Source: CAD feature listing. Evaluate the final solid. Frame: model axes, mm. A direction names the side the tool comes from. Coordinates: 2 decimals unless noted, no trailing zeros. Write each loop counter-clockwise with the first axis right and the second up, starting at its lowest first coordinate (ties: lowest second). Pieces come first, ordered by that corner, then holes. Notation, with made-up numbers: (43, 61) - (52, 61) arc R28 cw to (52, 89) - close; hole circle Ø1 at (24, 78.25). An arc over 180 degrees is marked (long way). One line per item, written item: value.
Autodesk Inventor part; units mm, degrees
ref_plane "Work Plane6" through (4.5, 0, 0) normal (1, 0, 0) x (0, 1, 0)
ref_plane "Work Plane7" through (0, -17.5, 0) normal (0, 1, 0) x (-1, 0, 0)
ref_plane "Work Plane8" through (0, 0, 15.25) normal (0, 0, 1) x (1, 0, 0)
sketch "Sketch1" plane through (0, 0, 0) normal (0, 0, 1) x (1, 0, 0)
  line L0 (-41.267, 50.1755) -> (50.733, 50.1755)
  line L1 (50.733, 50.1755) -> (50.733, -91.8245)
  line L2 (50.733, -91.8245) -> (-41.267, -91.8245)
  line L3 (-41.267, -91.8245) -> (-41.267, 50.1755)
  point P0 (0, 0)
  dimension "d0" = 142
  dimension "d1" = 92
extrude "Extrusion1" add sketch "Sketch1" along normal blind 14
sketch "Sketch2" plane through (0, 0, 14) normal (0, 0, 1) x (1, 0, 0)
  line L0 (50.733, 50.1755) -> (-41.267, 50.1755)
  line L1 (-41.267, -91.8245) -> (50.733, -91.8245)
  line L2 (50.733, -91.8245) -> (50.733, 50.1755)
  line L3 (50.733, 50.1755) -> (-41.267, 50.1755)
  line L4 (-41.267, 50.1755) -> (-41.267, -91.8245)
  circle A0 centre (29.733, 34.3976) radius 9
  circle A1 centre (-20.267, 34.3976) radius 9
  circle A2 centre (-20.267, -65.6024) radius 9
  circle A3 centre (29.733, -65.6024) radius 9
  point P0 (0, 0)
  point P1 (-20.267, 50.1755)
  point P2 (29.733, 50.1755)
  point P3 (50.733, 29.1755)
  point P4 (-41.267, 29.1755)
  point P5 (-41.267, 29.1755)
  point P6 (-20.267, 50.1755)
  point P7 (50.733, 29.1755)
  dimension "d5" = 21
  dimension "d6" = 21
  dimension "d7" = 50
  dimension "d8" = 21
  dimension "d9" = 21
  dimension "d13" = 18
  dimension "d14" = 18
  dimension "d15" = 100
  dimension "d16" = 100
  dimension "d17" = 18
  dimension "d18" = 18
extrude "Extrusion2" cut sketch "Sketch2" against normal through all contours A0 | A1 | A2 | A3
sketch "Sketch3" plane through (0, 0, 14) normal (0, 0, 1) x (1, 0, 0)
  circle A0 centre (-20.267, 34.3976) radius 9
  circle A1 centre (29.733, 34.3976) radius 9
  line L0 (50.733, -91.8245) -> (50.733, 50.1755)
  line L1 (-41.267, 50.1755) -> (-41.267, -91.8245)
  line L2 (50.733, -8.1024) -> (-41.267, -8.1024)
  line L3 (-41.267, -8.1024) -> (-41.267, -26.6259)
  line L4 (-41.267, -26.6259) -> (50.733, -26.6259)
  line L5 (50.733, -26.6259) -> (50.733, -8.1024)
  point P0 (0, 0)
  point P1 (-20.267, -8.1024)
  point P2 (31.8821, -8.1024)
  point P3 (50.733, -81.8245)
  point P4 (50.733, 40.1755)
  point P5 (-41.267, 40.1755)
  point P6 (-41.267, -81.8245)
  dimension "d22" = 42.5
  dimension "d23" = 42.5
  dimension "d54" = 92
  dimension "d55" = 92
extrude "Extrusion5" add sketch "Sketch3" along normal blind 58 contours L4 L1 L2 L0
chamfer "Chamfer1" distance 36 angle 45 2 edges at (50.733, -17.3641, 72) (-41.267, -17.3641, 72)
sketch "Sketch10" plane through (-41.267, -8.1024, 14) normal (0, 1, 0) x (1, 0, 0)
  line L0 (92, 0) -> (92, -22)
  line L1 (0, 0) -> (92, 0)
  point P0 (41.267, 14)
sketch "Sketch11" plane through (-41.267, -26.6259, 14) normal (0, -1, 0) x (1, 0, 0)
  line L0 (92, 0) -> (0, 0)
  line L1 (36, 58) -> (56, 58)
  point P0 (41.267, -14)
  point P1 (46, 58)
  point P2 (46, 0)
  dimension "d64" = 46
  dimension "d65" = 46
ref_plane "Work Plane6" through (4.5, 0, 0) normal (1, 0, 0) x (0, 1, 0)
sketch "Sketch12" plane through (4.5, 0, 0) normal (1, 0, 0) x (0, 1, 0)
  line L0 (-8.1024, 14) -> (32.8976, 14)
  line L1 (-8.1024, 14) -> (-8.1024, 72)
  line L2 (-8.1024, 72) -> (32.8976, 14)
  line L3 (-26.6259, 14) -> (-67.6259, 14)
  line L4 (-67.6259, 14) -> (-26.6259, 72)
  line L5 (-26.6259, 72) -> (-26.6259, 14)
  point P0 (0, 0)
  dimension "d67" = 41
  dimension "d68" = 41
extrude "Extrusion6" add sketch "Sketch12" along normal mid plane 15
sketch "Sketch13" plane through (0, 0, 0) normal (0, 1, 0) x (-1, 0, 0)
  point P0 (0, 0)
ref_plane "Work Plane7" through (0, -17.5, 0) normal (0, 1, 0) x (-1, 0, 0)
sketch "Sketch14" plane through (0, -17.5, 0) normal (0, 1, 0) x (-1, 0, 0)
  line L0 (3, 72) -> (-12, 72)
  circle A0 centre (-4.5, 72) radius 27.5
  circle A1 centre (-4.5, 72) radius 15
  point P0 (0, 0)
  dimension "d72" = 55
  dimension "d73" = 30
extrude "Extrusion7" add sketch "Sketch14" along normal mid plane 45
ref_plane "Work Plane8" through (0, 0, 15.25) normal (0, 0, 1) x (1, 0, 0)
sketch "Sketch18" plane through (0, 0, 15.25) normal (0, 0, 1) x (1, 0, 0)
  line L0 (-41.267, 50.1755) -> (-41.267, -91.8245)
  point P0 (0, 0)
  point P1 (-41.267, -16.0035)
  dimension "d77" = 66.179
  dimension "d78" = 75.821
sketch "Sketch19" plane through (0, 5, 0) normal (0, 1, 0) x (1, 0, 0)
  circle A0 centre (4.5, -72) radius 15
  point P0 (0, 0)
extrude "Extrusion8" cut sketch "Sketch19" against normal blind 45
fillet "Fillet3" radius 10 4 edges at (50.733, -91.8245, 7) (-41.267, 50.1755, 7) (50.733, 50.1755, 7) (-41.267, -91.8245, 7)
properties material "Nickel-Copper Alloy 400"
1) Section query C-C on x = 35. Output: boundary loops of the cut face in (y, z).
Values found:
outline: (-91.82, 0) - (-72.9, 0) - (-72.9, 14) - (-91.82, 14) - close; (-58.3, 0) - (27.1, 0) - (27.1, 14) - (-8.1, 14) - (-8.1, 51.73) - (-26.63, 51.73) - (-26.63, 14) - (-58.3, 14) - close; (41.7, 0) - (50.18, 0) - (50.18, 14) - (41.7, 14) - close
2) Reachability of faces 1 (the flat face through (12, -43, 29)), 2 (the flat face through (-22, -8.102, 31)), 3 (the flat face through (-22, -26.626, 31)) from +Z, -Z, +X, -X, +Y, -Y: full face, straight path, thin tool, end or side. Return the list, or none.
Values found:
face 1: +X, -Y
face 2: -X, +Y
face 3: -X, -Y
3) Section query D-D on z = 21.5. Output: boundary loops of the cut face in (x, y).
Values found:
outline: (-41.27, -26.63) - (-3, -26.63) - (-3, -62.32) - (12, -62.32) - (12, -26.63) - (50.73, -26.63) - (50.73, -8.1) - (12, -8.1) - (12, 27.6) - (-3, 27.6) - (-3, -8.1) - (-41.27, -8.1) - close
4) Section query A-A on x = 4.5. Output: boundary loops of the cut face in (y, z).
Values found:
outline: (-91.82, 0) - (50.18, 0) - (50.18, 14) - (32.9, 14) - (5, 53.46) - (5, 57) - (-40, 57) - (-40, 53.08) - (-67.63, 14) - (-91.82, 14) - close; (-40, 87) - (5, 87) - (5, 99.5) - (-40, 99.5) - close
5) Draft query along Z for faces 4 (the flat face through (12, 8, 30)), 5 (the flat face through (4.395, -54.006, 33.267)), 6 (the flat face through (5, -91.824, 7)), 7 (the flat face through (-3, -43, 29)). Return one class per face: released by +Z, released by -Z, zero draft, split by the parting line, or undercut.
Values found:
face 4: undercut
face 5: released by +Z
face 6: zero draft
face 7: undercut
6) Contact query for flat-ended pins moving along their axis: P1, Ø6, axis at x = 21.5, y = -25, coming from the +Z side; P2, Ø11.5, axis at x = 25, z = 31.5, coming from the +Y side; P3, Ø17.5, axis at x = 4.5, y = 22.5, coming from the +Z side. Output: stop coordinate, or through.
Values found:
P1: z = 95.67
P2: y = -8.1
P3: z = 41.09
7) Material intervals for line 1 (Y direction, x = 30, z = 11); line 2 (X direction, y = -13.5, z = 72.5); line 3 (Y direction, x = -25.5, z = 18), sorted ascending.
Values found:
line 1: -91.82 to -74.6, -56.61 to 25.4, 43.39 to 50.18
line 2: -23 to -10.49, 19.49 to 32
line 3: -26.63 to -8.1
8) Section query B-B on z = 84. Output: boundary loops of the cut face in (x, y).
Values found:
outline: (-20.24, -40) - (-4.5, -40) - (-4.5, 5) - (-20.24, 5) - close; (13.5, -40) - (29.24, -40) - (29.24, 5) - (13.5, 5) - close
